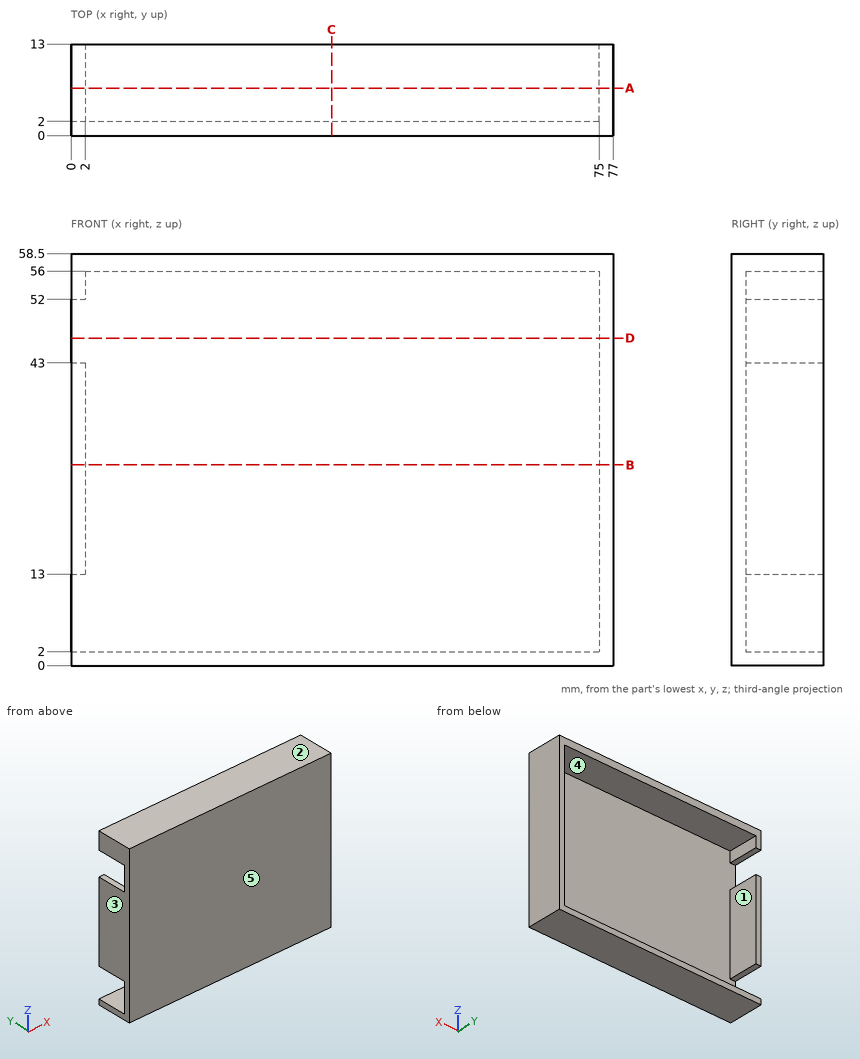
The figure shows three views and two pictorial views of one solid part (mm, origin at its lowest corner). Answer the questions. A direction names the side the tool comes from. Give positions to 0.01 mm unless a question says otherwise; leave off trailing zeros. Write each loop counter-clockwise with the first axis right and the second up, starting at its lowest first coordinate (ties: lowest second). Pieces come first, ordered by that corner, then holes. Notation, with made-up numbers: (28.25, -7.5) - (43.25, -7.5) arc R24 cw to (43.25, 6.5) - close; hole circle Ø9 at (83.25, 54). An arc over 180 degrees is marked (long way). Return JSON: item names as keys, results as strings.
Q1. A cutting plane is placed at B-B, the plane z = 28.5. Determine the outline of the cut face in (x, y), and give its area (3 significant figures).
Reply:
{"outline": "(0, 0) - (77, 0) - (77, 13) - (75, 13) - (75, 2) - (2, 2) - (2, 13) - (0, 13) - close", "area": "198 mm²"}
Q2. For the marked faces 1 and 2, determine the directions among +Z, -Z, +X, -X, +Y, -Y from which every point of the face is accessible in a straight line to the end or side of a thin tool.
Reply:
{"face 1": "+Y", "face 2": "+Z, +X, -X, +Y, -Y"}
Q3. For a pull along X with two mould halves and no side action, classify the marked faces 3, 4 and 5 as released by +X, released by -X, zero draft, split by the parting line, or undercut.
Reply:
{"face 3": "released by -X", "face 4": "undercut", "face 5": "zero draft"}
Q4. Given P1, Ø2, axis at x = 67.5, y = 5, coming from the -Z side; P2, Ø6, axis at x = 47.5, z = 24, coming from the +Y side, each flat-ended and moving along its own axis, determine where each tip first touches the part or whether it passes through.
Reply:
{"P1": "z = 0", "P2": "y = 2"}
Q5. A cutting plane is placed at D-D, the plane z = 46.5. Determine the outline of the cut face in (x, y).
Reply:
{"outline": "(0, 0) - (77, 0) - (77, 13) - (75, 13) - (75, 2) - (0, 2) - close"}
Q6. Consider line 1 along X through (y, z) = (3.75, 55.5); line 2 along Z through (x, y) = (48.5, 4.5); line 3 along Y through (x, z) = (24.5, 37). Determine where each line is inside the solid, lowest interval first. Write a range as [from, to].
Reply:
{"line 1": "[0, 2], [75, 77]", "line 2": "[0, 2], [56, 58.5]", "line 3": "[0, 2]"}
Q7. A cutting plane is placed at A-A, the plane y = 6.75. Determine the outline of the cut face in (x, z), and give its area (4 significant figures).
Reply:
{"outline": "(0, 0) - (77, 0) - (77, 58.5) - (0, 58.5) - (0, 52) - (2, 52) - (2, 56) - (75, 56) - (75, 2) - (0, 2) - close; (0, 13) - (2, 13) - (2, 43) - (0, 43) - close", "area": "522.5 mm²"}
Q8. A cutting plane is placed at C-C, the plane x = 37. Determine the outline of the cut face in (y, z).
Reply:
{"outline": "(0, 0) - (13, 0) - (13, 2) - (2, 2) - (2, 56) - (13, 56) - (13, 58.5) - (0, 58.5) - close"}
